Could you check a few things on this model? Use its own coordinates, in mm. A direction names the side the tool comes from. Give positions to 0.01 mm unless a question says otherwise; leave off trailing zeros. Loops run counter-clockwise (first coordinate to the right, second up) from the corner with the lowest first, then second, coordinate; pieces in that order, holes last. Notation, with made-up numbers: M 77,-14.5 L 107,-14.5 A13 cw 107,8.5 Z; hole C -17,62.5 d7. An arc over 180 degrees is marked long. Use a Markdown table: item, result. Add a question column.
1) Suppose I cut it at B-B on x = 0. List the corners of the cut face in (y, z) for me.
2) We'd pull the mould along X, two halves only. Please class faces 1 (the flat face through (14.364, 11.471, 4.93)), 2 (the flat face through (-14.603, 11.375, 4.93)), 3 (the flat face through (2, -6, 14)), 4 (the cylindrical face through (6, 0, 20)): +X half, -X half, draft (parallel to the pull), parting line (faces both ways), or undercut.
3) Suppose I cut it at A-A on y = 0. Count the separate pieces of the cut face and the enclosed holes in it, and give its area (3 significant figures).
4) Will these pins go through, and if not, where does the flat tip stop? pin 1 Ø4 at (x, z) = (-23, 8) entering from +Y; pin 2 Ø7 at (x, y) = (0, 0) entering from -Z; pin 3 Ø1 at (x, z) = (23, 6.5) entering from -Y; pin 4 Ø8 at (y, z) = (6, 7) entering from -X.
5) If I drill on line 1 along Y through (x, z) = (0, 19); line 2 along Y through (x, z) = (23, 2.75); line 3 along X through (y, z) = (3.5, 8), over which ranges is the centre line in solid material (lowest first)? Write a range as [from, to].
6) Which directions (+Z, -Z, +X, -X, +Y, -Y) give clear straight access to the entire face, cutting with the end or side of a thin tool? Please do faces 5 (the cylindrical face through (-31, 0, 5)), 6 (the cylindrical face through (-2.38, -10.74, 17.92)).
7) Suppose I cut it at C-C on z = 9. List the corners of the cut face in (x, y) for me.
8) Suppose I cut it at D-D on x = 20. List the corners of the cut face in (y, z) for me.
```python
from build123d import *

# Parameters (mm, degrees)
SKETCH_1_R      = 4.5
EXTRUDE_1_DEPTH = 10
SKETCH_4_R      = 11
EXTRUDE_2_DEPTH = 25
FILLET_1_R      = 2
CHAMFER_1_SIZE  = 1


with BuildPart() as part:
    # Эскиз1 → Бобышка-Вытянуть1 (new body)
    with BuildSketch(Plane.XY):
        with BuildLine():
            Line((-23, 8), (-5.966665012, 14.845838091))
            ThreePointArc((-5.966665012, 14.845838091), (0, 16), (5.966665012, 14.845838091))
            Line((5.966665012, 14.845838091), (23, 8))
            ThreePointArc((23, 8), (31, 0), (23, -8))
            Line((23, -8), (5.966665012, -14.845838091))
            ThreePointArc((5.966665012, -14.845838091), (0, -16), (-5.966665012, -14.845838091))
            Line((-5.966665012, -14.845838091), (-23, -8))
            ThreePointArc((-23, -8), (-31, 0), (-23, 8))
        make_face()
        with Locations((-23, 0)):
            Circle(SKETCH_1_R, mode=Mode.SUBTRACT)
        with Locations(Location((23, 0, 0), (0, 0, 180))):
            Circle(SKETCH_1_R, mode=Mode.SUBTRACT)
    extrude(amount=EXTRUDE_1_DEPTH)

    # Эскиз4 → Бобышка-Вытянуть2 (add)
    with BuildSketch(Plane.XY):
        Circle(SKETCH_4_R)
    extrude(amount=EXTRUDE_2_DEPTH)

    # Эскиз5 → Вырез-Повернуть1 (revolve, cut)
    with BuildSketch(Plane(origin=(0, 0, 0), x_dir=(1, 0, 0), z_dir=(0, 1, 0))):
        with BuildLine():
            Line((0, 0), (-10, 0))
            Line((-10, 0), (-8.122654092, -13.141421356))
            ThreePointArc((-8.122654092, -13.141421356), (-7.78790634, -13.755453955), (-7.132704598, -14))
            Line((-7.132704598, -14), (-6, -14))
            Line((-6, -14), (-6, -25))
            Line((-6, -25), (0, -25))
            Line((0, -25), (0, 0))
        make_face()
    revolve(axis=Axis((0, 0, -38.345280775), (0, 0, 1)), mode=Mode.SUBTRACT)

    # Скругление1
    fillet_1_edges = [part.edges().sort_by_distance(p)[0] for p in [
        (-11, 0, 10),
    ]]
    fillet(fillet_1_edges, radius=FILLET_1_R)

    # Фаска1
    chamfer_1_edges = [part.edges().sort_by_distance(p)[0] for p in [
        (-11, 0, 25),
    ]]
    chamfer(chamfer_1_edges, length=CHAMFER_1_SIZE)


solid = part.part
```
Answer block:
| question | item | result |
|---|---|---|
| 1 | outline | M -16,0 L -10,0 L -8.12,13.14 A1 cw -7.13,14 L -6,14 L -6,25 L -10,25 L -11,24 L -11,12 A2 cw -13,10 L -16,10 Z; M 6,14 L 7.13,14 A1 cw 8.12,13.14 L 10,0 L 16,0 L 16,10 L 13,10 A2 cw 11,12 L 11,24 L 10,25 L 6,25 Z |
| 2 | face 1 | +X half |
| 2 | face 2 | -X half |
| 2 | face 3 | undercut |
| 2 | face 4 | undercut |
| 3 | separate pieces | 4 |
| 3 | enclosed holes | 0 |
| 3 | area | 387 mm^2 |
| 4 | pin 1 | stops at y = 8.8 |
| 4 | pin 2 | passes through |
| 4 | pin 3 | stops at y = -8.2 |
| 4 | pin 4 | stops at x = -30.75 |
| 5 | line 1 | y = [-11, -6], [6, 11] |
| 5 | line 2 | y = [-8, -4.5], [4.5, 8] |
| 5 | line 3 | x = [-30.19, -25.83], [-20.17, -8.14], [8.14, 20.17], [25.83, 30.19] |
| 6 | face 5 | +Z, -Z, -X |
| 6 | face 6 | +Z |
| 7 | outline | M -23,-8 L -5.97,-14.85 A16 ccw 5.97,-14.85 L 23,-8 A8 ccw 23,8 L 5.97,14.85 A16 ccw -5.97,14.85 L -23,8 A8 ccw Z; hole C -23,0 d9; hole C 0,0 d17.43; hole C 23,0 d9 |
| 8 | outline | M -9.21,0 L -3.35,0 L -3.35,10 L -9.21,10 Z; M 3.35,0 L 9.21,0 L 9.21,10 L 3.35,10 Z |
